The listing builds one solid part. Answer for the finished solid, in the listing's coordinates (mm). A direction names the side the tool comes from. Give positions to 0.01 mm unless a question says otherwise; leave off trailing zeros. Answer as a JSON object with one key per item and string values. Group by question number.
```python
from build123d import *

# Parameters (mm, degrees)
SKETCH1_W                      = 12
SKETCH1_H                      = 8
BOSS_EXTRUDE1_DEPTH            = 400
CBORE_FOR_M3_SHCS1_D           = 3.4
CBORE_FOR_M3_SHCS1_CBORE_D     = 6.5
CBORE_FOR_M3_SHCS1_CBORE_DEPTH = 4.5
LPATTERN1_COUNT                = 16
LPATTERN1_PITCH                = 25


with BuildPart() as part:
    # Sketch1 → Boss-Extrude1 (new body)
    with BuildSketch(Plane.XY):
        with Locations((6, 4)):
            Rectangle(SKETCH1_W, SKETCH1_H)
    extrude(amount=BOSS_EXTRUDE1_DEPTH)

    # CBORE for M3 SHCS1 (through all)
    with Locations(Plane(origin=(0, 8, 0), x_dir=(1, 0, 0), z_dir=(0, 1, 0))):
        with Locations((6, -387.5)):
            cbore_for_m3_shcs1 = CounterBoreHole(CBORE_FOR_M3_SHCS1_D / 2, CBORE_FOR_M3_SHCS1_CBORE_D / 2, CBORE_FOR_M3_SHCS1_CBORE_DEPTH)

    # LPattern1: CBORE for M3 SHCS1 ×16
    with Locations(*[(0, 0, -i * LPATTERN1_PITCH) for i in range(1, LPATTERN1_COUNT)]):
        add(cbore_for_m3_shcs1, mode=Mode.SUBTRACT)


solid = part.part
```
Item 1: Flat-ended cylindrical pins translate along their axes: P1, Ø2, axis at x = 6, z = 212.5, coming from the +Y side; P2, Ø6, axis at x = 6, z = 262.5, coming from the +Y side. Find the tip coordinate at first contact, or state that the pin passes through.
Item 2: Determine the mould class of faces 1 (the cylindrical face through (7.75, 5.78, 9.76)), 2 (the flat face through (6, 4, 400)), 3 (the flat face through (0, 4, 197)) for opening direction Z: released by +Z, released by -Z, zero draft, split by the parting line, or undercut.
Item 3: A tool of negligible diameter and unlimited length cuts with its end or side. For faces 4 (the flat face through (6, 8, 197)), 5 (the flat face through (7.4, 3.5, 88.9)), from which of +Z, -Z, +X, -X, +Y, -Y can it reach the whole face along a straight path? Write none if from no direction.
Item 4: Consider probe 1 along X at (y, z) = (3.25, 88); probe 2 along X at (y, z) = (1.35, 112.5). Determine where each line is inside the solid, lowest interval first. Write a range as from..to.
Item 5: Section A-A (y = 1.75) is taken. Count the separate pieces of the cut face and the enclosed holes in it, and give its area (3 significant figures).
Values found:
{
 "1": {"P1": "passes through", "P2": "stops at y = 3.5"},
 "2": {"face 1": "undercut", "face 2": "released by +Z", "face 3": "zero draft"},
 "3": {"face 4": "+Z, -Z, +X, -X, +Y", "face 5": "+Y"},
 "4": {"probe 1": "x = 0..4.38, 7.62..12", "probe 2": "x = 0..4.3, 7.7..12"},
 "5": {"separate pieces": "1", "enclosed holes": "16", "area": "4,650 mm^2"}
}
